The listing builds one solid part. Answer for the finished solid, in the listing's coordinates (mm). Face numbers are marked on the shaded views. A direction names the side the tool comes from. Coordinates: 2 decimals unless noted, no trailing zeros. Order: outer loops, then holes, each group sorted by start corner. A loop starts at its lowest first (then second) coordinate and runs counter-clockwise, first axis right, second up. Notation, with made-up numbers: (67, 28) - (93, 28) arc R21 ccw to (93, 43) - close; hole circle Ø6 at (78, -18.75). An arc over 180 degrees is marked (long way). Use a Markdown table: item, result. Add a question column.
Item 1: For the marked faces 1, 2 and 3, determine the directions among +Z, -Z, +X, -X, +Y, -Y from which every point of the face is accessible in a straight line to the end or side of a thin tool.
Item 2: Find the intervals of material crossed by line 1 along X through (y, z) = (6.4, 3.5); line 2 along Y through (x, z) = (0, -3.95); line 3 along Z through (x, y) = (26, 2.5), in increasing order.
Item 3: The part is cut by section D-D, the plane x = 0. Give the vertices of the cut face in (y, z), then the cut area to 3 significant figures.
Item 4: The part is cut by section B-B, the plane y = 1.75. State how many separate pieces and enclosed holes the cut face has, then the cut area to 3 significant figures.
Item 5: Flat-ended cylindrical pins translate along their axes: P1, Ø0.9, axis at x = -35, y = 2, coming from the -Z side; P2, Ø3, axis at x = 0, y = 15, coming from the +Z side; P3, Ø1.8, axis at x = -37, z = 3, coming from the -Y side. Find the tip coordinate at first contact, or state that the pin passes through.
Item 6: The part is cut by section A-A, the plane x = -36. Give the vertices of the cut face in (y, z).
Item 7: The part is cut by section C-C, the plane z = 25. Give the vertices of the cut face in (x, y).
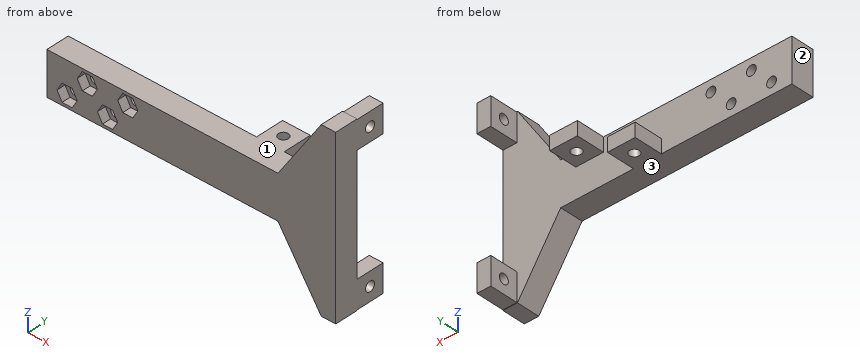
from build123d import *

# Parameters (mm, degrees)
BOSS_EXTRUDE1_DEPTH = 8
SKETCH2_W           = 4.8
SKETCH2_H           = 9.6
SKETCH2_W_2         = 9.6
SKETCH2_H_2         = 4.8
BOSS_EXTRUDE2_DEPTH = 9.8
CUT_EXTRUDE1_REACH  = 103.39
SKETCH3_R           = 1.7
CUT_EXTRUDE2_REACH  = 64.339
SKETCH4_R           = 1.7
CUT_EXTRUDE3_REACH  = 64.339
SKETCH5_R           = 1.7
CUT_EXTRUDE4_START  = -5
CUT_EXTRUDE4_DEPTH  = 3
SKETCH10_R          = 1.7
CUT_EXTRUDE7_DEPTH  = 5
LPATTERN2_COUNT     = 2
LPATTERN2_PITCH     = 14


with BuildPart() as part:
    # Sketch1 → Boss-Extrude1 (new body)
    with BuildSketch(Plane(origin=(0, 0, 0), x_dir=(1, 0, 0), z_dir=(0, 1, 0))):
        Polygon((50, 30), (50, -30), (45, -30), (30, -7.5), (-50, -7.5), (-50, 7.5), (30, 7.5), (45, 30), align=None)
    extrude(amount=BOSS_EXTRUDE1_DEPTH)

    # Sketch2 → Boss-Extrude2 (add)
    with BuildSketch(Plane(origin=(0, 8, 0), x_dir=(1, 0, 0), z_dir=(0, 1, 0))):
        with Locations((47.6, 25)):
            Rectangle(SKETCH2_W, SKETCH2_H)
        with Locations((47.6, -25)):
            Rectangle(SKETCH2_W, SKETCH2_H)
        with Locations((20, -5.1)):
            Rectangle(SKETCH2_W_2, SKETCH2_H_2)
        with Locations((0, 5.1)):
            Rectangle(SKETCH2_W_2, SKETCH2_H_2)
    extrude(amount=BOSS_EXTRUDE2_DEPTH)

    # Sketch3 → Cut-Extrude1 (cut, up to next)
    with BuildSketch(Plane.ZY.offset(-45.2), mode=Mode.PRIVATE) as cut_extrude1_sk1:
        with Locations((-25, 12.9)):
            Circle(SKETCH3_R)
    cut_extrude1_tool1 = extrude(cut_extrude1_sk1.sketch, amount=-CUT_EXTRUDE1_REACH, mode=Mode.PRIVATE) & part.part
    cut_extrude1 = cut_extrude1_tool1.solids().sort_by_distance((45.2, 12.9, -25))[0]
    add(cut_extrude1, mode=Mode.SUBTRACT)

    # Mirror1: Cut-Extrude1 across plane
    add(cut_extrude1.mirror(Plane.XY), mode=Mode.SUBTRACT)

    # Sketch4 → Cut-Extrude2 (cut, up to next)
    with BuildSketch(Plane(origin=(0, 0, 2.7), x_dir=(-1, 0, 0), z_dir=(0, 0, -1)), mode=Mode.PRIVATE) as cut_extrude2_sk1:
        with Locations((-20, 12.9)):
            Circle(SKETCH4_R)
    cut_extrude2_tool1 = extrude(cut_extrude2_sk1.sketch, amount=-CUT_EXTRUDE2_REACH, mode=Mode.PRIVATE) & part.part
    add(cut_extrude2_tool1.solids().sort_by_distance((20, 12.9, 2.7))[0], mode=Mode.SUBTRACT)

    # Sketch5 → Cut-Extrude3 (cut, up to next)
    with BuildSketch(Plane.XY.offset(-2.7), mode=Mode.PRIVATE) as cut_extrude3_sk1:
        with Locations((0, 12.9)):
            Circle(SKETCH5_R)
    cut_extrude3_tool1 = extrude(cut_extrude3_sk1.sketch, amount=-CUT_EXTRUDE3_REACH, mode=Mode.PRIVATE) & part.part
    add(cut_extrude3_tool1.solids().sort_by_distance((0, 12.9, -2.7))[0], mode=Mode.SUBTRACT)

    # Sketch7 → Cut-Extrude4 (cut)
    with BuildSketch(Plane(origin=(0, 8, 0), x_dir=(1, 0, 0), z_dir=(0, 1, 0)).offset(CUT_EXTRUDE4_START)):
        Polygon((-46.5, 3.5), (-44.75, 0.468911087), (-41.25, 0.468911087), (-39.5, 3.5), (-41.25, 6.531088913), (-44.75, 6.531088913), align=None)
        Polygon((-32.5, -3.5), (-34.25, -0.468911087), (-37.75, -0.468911087), (-39.5, -3.5), (-37.75, -6.531088913), (-34.25, -6.531088913), align=None)
    cut_extrude4 = extrude(amount=-CUT_EXTRUDE4_DEPTH, mode=Mode.SUBTRACT)

    # Sketch10 → Cut-Extrude7 (cut)
    with BuildSketch(Plane.XZ.offset(-3)):
        with Locations(Location((-43, -3.5, 0), (0, 0, 270))):
            Circle(SKETCH10_R)
        with Locations(Location((-36, 3.5, 0), (0, 0, 270))):
            Circle(SKETCH10_R)
    cut_extrude7 = extrude(amount=-CUT_EXTRUDE7_DEPTH, mode=Mode.SUBTRACT)

    # LPattern2: Cut-Extrude4, Cut-Extrude7 ×2
    with Locations(*[(i * LPATTERN2_PITCH, 0, 0) for i in range(1, LPATTERN2_COUNT)]):
        add(cut_extrude4, mode=Mode.SUBTRACT)
        add(cut_extrude7, mode=Mode.SUBTRACT)


solid = part.part
Solution:
| question | item | result |
|---|---|---|
| 1 | face 1 | +Z, -X, +Y, -Y |
| 1 | face 2 | +Z, -Z, -X, +Y, -Y |
| 1 | face 3 | -Z, -X, +Y, -Y |
| 2 | line 1 | x = -50 to -37.7, -34.3 to -23.7, -20.3 to 50 |
| 2 | line 2 | y = 0 to 11.2, 14.6 to 17.8 |
| 2 | line 3 | z = -7.5 to 7.5 |
| 3 | outline | (0, -7.5) - (11.2, -7.5) - (11.2, -2.7) - (8, -2.7) - (8, 7.5) - (0, 7.5) - close; (14.6, -7.5) - (17.8, -7.5) - (17.8, -2.7) - (14.6, -2.7) - close |
| 3 | area | 151 mm2 |
| 4 | separate pieces | 1 |
| 4 | enclosed holes | 4 |
| 4 | area | 1,940 mm2 |
| 5 | P1 | stops at z = -7.5 |
| 5 | P2 | stops at z = -2.7 |
| 5 | P3 | stops at y = 3 |
| 6 | outline | (0, -7.5) - (8, -7.5) - (8, 1.8) - (3, 1.8) - (3, 0.47) - (0, 0.47) - close; (0, 6.53) - (3, 6.53) - (3, 5.2) - (8, 5.2) - (8, 7.5) - (0, 7.5) - close |
| 7 | outline | (41.67, 0) - (50, 0) - (50, 11.2) - (45.2, 11.2) - (45.2, 8) - (41.67, 8) - close; (45.2, 14.6) - (50, 14.6) - (50, 17.8) - (45.2, 17.8) - close |
